Drawing for the job (mm, zero at the part's lowest x, y, z). A direction names the side the tool comes from. Round coordinates to 2 decimals unless told otherwise and drop trailing zeros. Write each loop counter-clockwise with the first axis right and the second up, starting at its lowest first coordinate (ties: lowest second). Pieces come first, ordered by that corner, then holes. Notation, with made-up numbers: (11.25, 58) - (39.25, 58) arc R22 cw to (39.25, 83) - close; hole circle Ø3 at (30, 20.5). An arc over 180 degrees is marked (long way). One line per question, with ' | ' between items.
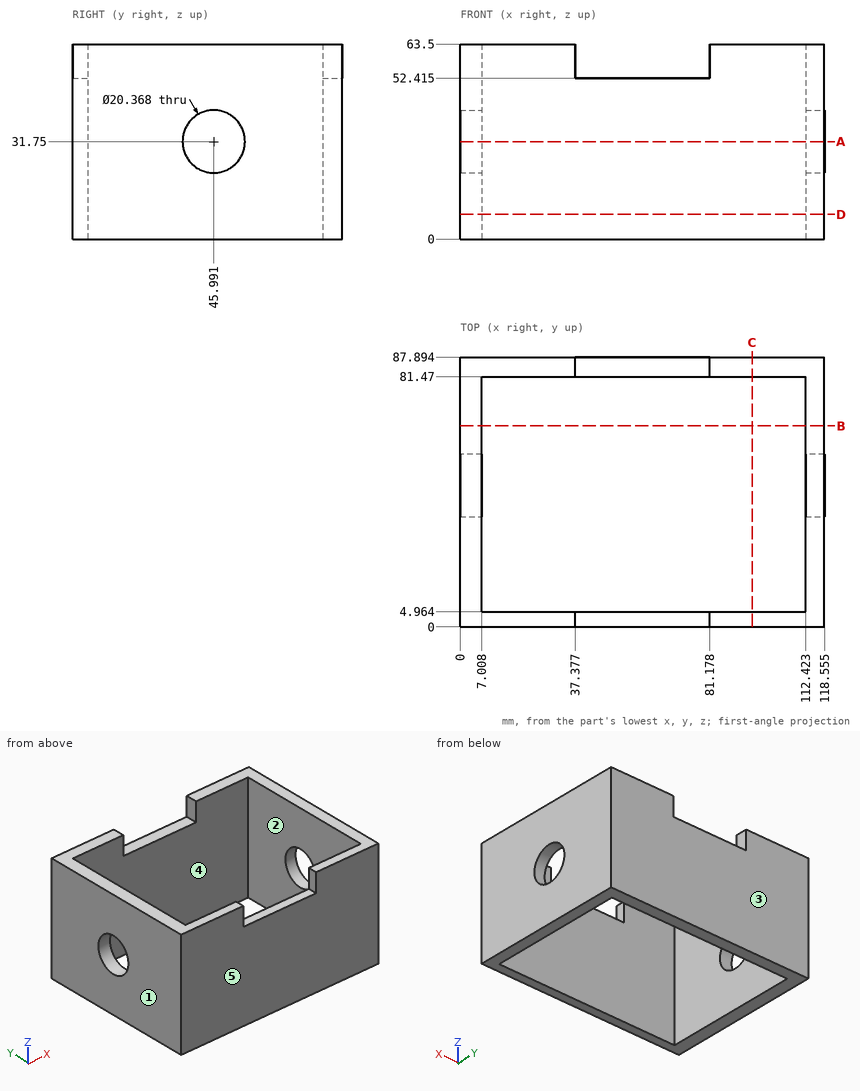
Q1. Saw through at A-A, the plane z = 31.75. List the corners of the cut face in (x, y) (1 decimal).
Found:
outline: (0, 0) - (118.6, 0) - (118.6, 35.8) - (112.4, 35.8) - (112.4, 5) - (7, 5) - (7, 35.8) - (0, 35.8) - close; (0, 56.2) - (7, 56.2) - (7, 81.5) - (112.4, 81.5) - (112.4, 56.2) - (118.6, 56.2) - (118.6, 87.9) - (0, 87.9) - close
Q2. Pull direction Y, two halves, no side cores. Call the marked faces 3, 4 and 5: +Y half, -Y half, draft (parallel to the pull), parting line (faces both ways), or undercut.
Found:
face 3: +Y half | face 4: undercut | face 5: -Y half
Q3. Saw through at C-C, the plane x = 95. List the corners of the cut face in (y, z).
Found:
outline: (0, 0) - (4.96, 0) - (4.96, 63.5) - (0, 63.5) - close; (81.47, 0) - (87.89, 0) - (87.89, 63.5) - (81.47, 63.5) - close
Q4. Saw through at B-B, the plane y = 65.5. List the corners of the cut face in (x, z) (1 decimal).
Found:
outline: (0, 0) - (7, 0) - (7, 63.5) - (0, 63.5) - close; (112.4, 0) - (118.6, 0) - (118.6, 63.5) - (112.4, 63.5) - close
Q5. Which spindle directions (+Z, -Z, +X, -X, +Y, -Y) get a long thin tool onto all of the face, cutting with end or side? Do the marked faces 1 and 2. Say none if no direction does.
Found:
face 1: +Z, -Z, -X, +Y, -Y | face 2: +Z, -Z
Q6. Drop flat-ended pins along their axis: pin 1 (1.9 mm diameter, centred on x = 59.5, y = 84, fed in from +Z) (1 decimal); pin 2 (18.5 mm diameter, centred on y = 45.99, z = 31.75, fed in from -X). Give the stop position or say it passes through.
Found:
pin 1: z = 52.4 | pin 2: through
Q7. Saw through at D-D, the plane z = 8. List the corners of the cut face in (x, y) (1 decimal).
Found:
outline: (0, 0) - (118.6, 0) - (118.6, 87.9) - (0, 87.9) - close; hole (7, 5) - (112.4, 5) - (112.4, 81.5) - (7, 81.5) - close
Q8. Drill centre lines: L1, parallel to X at y = 44.5, z = 11 (1 decimal); L2, parallel to Y at x = 55, z = 10; L3, parallel to X at y = 4, z = 60 (1 decimal). Where is each one in solid material? Low to high. Write a range as from..to.
Found:
L1: 0..7, 112.4..118.6 | L2: 0..4.96, 81.47..87.89 | L3: 0..37.4, 81.2..118.6
